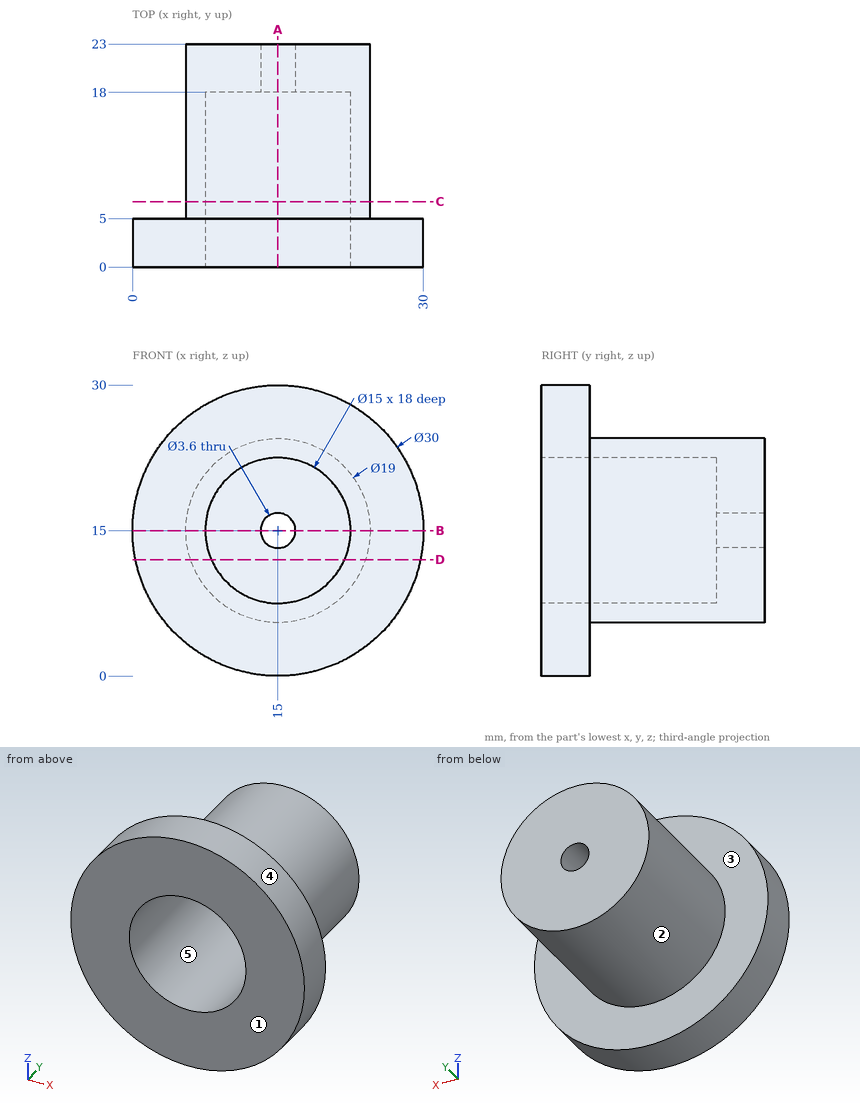
Geometry check sheet. Reference: drawing and pictorial views, mm from the part's lowest x, y, z. A direction names the side the tool comes from. Coordinates: 2 decimals unless noted, no trailing zeros. Loops run counter-clockwise (first coordinate to the right, second up) from the corner with the lowest first, then second, coordinate; pieces in that order, holes last. Notation, with made-up numbers: (20, -18) - (27, -18) arc R22 cw to (27, 1) - close; hole circle Ø2 at (-17.5, 19.25). An arc over 180 degrees is marked (long way). Return JSON: item names as keys, results as strings.
1. Thickness scan on L1, parallel to Z at x = 15, y = 14.25; L2, parallel to Z at x = 15, y = 19.95; L3, parallel to Y at x = 17.25, z = 10.25. Record the ranges inside material, lowest first.
Established:
{"L1": "z = 5.5 to 7.5, 22.5 to 24.5", "L2": "z = 5.5 to 13.2, 16.8 to 24.5", "L3": "y = 18 to 23"}
2. Tool access check on the marked faces 1 and 2. Record the directions out of +Z, -Z, +X, -X, +Y, -Y that give a thin tool (end or side, any length) a straight path to the whole face; none if there is none.
Established:
{"face 1": "+Z, -Z, +X, -X, -Y", "face 2": "+Y"}
3. Section check B-B, the plane z = 15. Record the boundary of the cut face in (x, y), then the cut area to 3 significant figures.
Established:
{"outline": "(0, 0) - (7.5, 0) - (7.5, 18) - (13.2, 18) - (13.2, 23) - (5.5, 23) - (5.5, 5) - (0, 5) - close; (16.8, 18) - (22.5, 18) - (22.5, 0) - (30, 0) - (30, 5) - (24.5, 5) - (24.5, 23) - (16.8, 23) - close", "area": "204 mm2"}
4. Section check C-C, the plane y = 6.75. Record the boundary of the cut face in (x, z).
Established:
{"outline": "circle Ø19 at (15, 15); hole circle Ø15 at (15, 15)"}
5. Go/stop test with flat-tipped pins: pin 1 (7.5 mm diameter, centred on x = 17, z = 16, fed in from -Y); pin 2 (8 mm diameter, centred on y = 17.5, z = 17.5, fed in from -X); pin 3 (2 mm diameter, centred on x = 4.5, z = 17.5, fed in from +Y). Record where each tip stops, or that it passes through.
Established:
{"pin 1": "stops at y = 18", "pin 2": "stops at x = 5.5", "pin 3": "stops at y = 5"}
6. Section check D-D, the plane z = 12. Record the boundary of the cut face in (x, y), then the cut area to 3 significant figures.
Established:
{"outline": "(0.3, 0) - (8.13, 0) - (8.13, 18) - (21.87, 18) - (21.87, 0) - (29.7, 0) - (29.7, 5) - (24.01, 5) - (24.01, 23) - (5.99, 23) - (5.99, 5) - (0.3, 5) - close", "area": "224 mm2"}
7. Mould release check, pull along X, two halves, no side actions. Record for the marked faces 3, 4 and 5: +X half, -X half, draft (parallel to the pull), parting line (faces both ways), or undercut.
Established:
{"face 3": "draft", "face 4": "parting line", "face 5": "undercut"}
8. Section check A-A, the plane x = 15. Record the boundary of the cut face in (y, z).
Established:
{"outline": "(0, 0) - (5, 0) - (5, 5.5) - (23, 5.5) - (23, 13.2) - (18, 13.2) - (18, 7.5) - (0, 7.5) - close; (0, 22.5) - (18, 22.5) - (18, 16.8) - (23, 16.8) - (23, 24.5) - (5, 24.5) - (5, 30) - (0, 30) - close"}
